Source: CAD feature listing. Evaluate the final solid. Frame: model axes, mm. Coordinates: 2 decimals unless noted, no trailing zeros. Write each loop counter-clockwise with the first axis right and the second up, starting at its lowest first coordinate (ties: lowest second). Pieces come first, ordered by that corner, then holes. Notation, with made-up numbers: M -3.5,-31 L 14.5,-31 A20 ccw 14.5,4 Z; hole C -7.5,85 d5. An arc over 180 degrees is marked long. Write item = value, one per line. Start each with the question number.
1. Section query A-A (y = 581). Output: boundary loops of the cut face in (x, z), then the cut area to 3 significant figures.
2. Section query C-C (x = 26.25). Output: boundary loops of the cut face in (y, z), then the cut area to 3 significant figures.
3. Pin query (flat end, axial travel): pin 1 Ø1.9 at (x, y) = (103.91, 584.08) entering from -Z. Return the tip coordinate at first contact, or that it passes through.
4. Line query: line 1 along X through (y, z) = (573.5, 0.65); line 2 along Y through (x, z) = (26.25, 1.25); line 3 along X through (y, z) = (570, 1.3). Output: solid intervals per line, ascending.
5. Section query D-D (z = 0.4). Output: boundary loops of the cut face in (x, y).
6. Section query B-B (x = 7). Output: boundary loops of the cut face in (y, z).
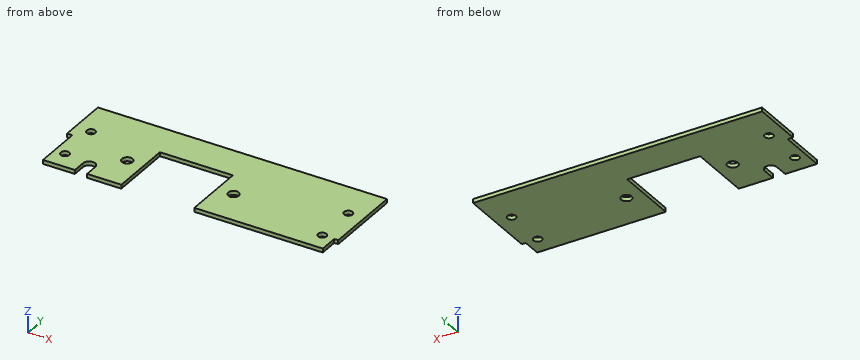
```python
from build123d import *

# Parameters (mm, degrees)
SKETCH1_W           = 110.914742868
SKETCH1_H           = 37
SKETCH1_R           = 1.6
BOSS_EXTRUDE1_DEPTH = 1.5
SKETCH2_W           = 3
SKETCH2_H           = 18
CUT_EXTRUDE1_DEPTH  = 1.5
SKETCH3_W           = 1.5
SKETCH3_H           = 7
SKETCH3_W_2         = 1
SKETCH3_H_2         = 30
SKETCH3_H_3         = 19
CUT_EXTRUDE2_DEPTH  = 10
SKETCH4_R           = 2
SKETCH4_W           = 27.5
SKETCH4_H           = 23.7
CUT_EXTRUDE3_DEPTH  = 10


with BuildPart() as part:
    # Sketch1 → Boss-Extrude1 (new body)
    with BuildSketch(Plane.XY):
        with Locations((55.457371434, 579.580871166)):
            Rectangle(SKETCH1_W, SKETCH1_H)
        with Locations((103.914742868, 584.080871166)):
            Circle(SKETCH1_R, mode=Mode.SUBTRACT)
        with Locations((103.914742868, 568.080871166)):
            Circle(SKETCH1_R, mode=Mode.SUBTRACT)
        with Locations((7, 584.080871166)):
            Circle(SKETCH1_R, mode=Mode.SUBTRACT)
        with Locations((7, 568.080871166)):
            Circle(SKETCH1_R, mode=Mode.SUBTRACT)
    extrude(amount=BOSS_EXTRUDE1_DEPTH)

    # Sketch2 → Cut-Extrude1 (cut)
    with BuildSketch(Plane.XY.offset(1.5)):
        with Locations((1.5, 570.080871166)):
            Rectangle(SKETCH2_W, SKETCH2_H)
    extrude(amount=-CUT_EXTRUDE1_DEPTH, mode=Mode.SUBTRACT)

    # Sketch3 → Cut-Extrude2 (cut)
    with BuildSketch(Plane.XY.offset(1.5)):
        with Locations((109.164742868, 564.580871166)):
            Rectangle(SKETCH3_W, SKETCH3_H)
        with Locations((110.414742868, 564.580871166)):
            Rectangle(SKETCH3_W_2, SKETCH3_H)
        with Locations((110.414742868, 583.080871166)):
            Rectangle(SKETCH3_W_2, SKETCH3_H_2)
        with Locations((0.5, 588.580871166)):
            Rectangle(SKETCH3_W_2, SKETCH3_H_3)
    extrude(amount=-CUT_EXTRUDE2_DEPTH, mode=Mode.SUBTRACT)

    # Sketch4 → Cut-Extrude3 (cut)
    with BuildSketch(Plane.XY.offset(1.5)):
        with Locations((66.25, 574.980871166)):
            Circle(SKETCH4_R)
        with Locations((26.25, 574.980871166)):
            Circle(SKETCH4_R)
        with Locations((46.25, 572.930871166)):
            Rectangle(SKETCH4_W, SKETCH4_H)
        with BuildLine():
            Line((15, 561.080871166), (15, 566.080871166))
            ThreePointArc((15, 566.080871166), (17.3, 568.380871166), (19.6, 566.080871166))
            Line((19.6, 566.080871166), (19.6, 561.080871166))
            ThreePointArc((19.6, 561.080871166), (17.3, 558.780871166), (15, 561.080871166))
        make_face()
    extrude(amount=-CUT_EXTRUDE3_DEPTH, mode=Mode.SUBTRACT)


solid = part.part
```
Results are:
q1.outline = M 1,0 L 32.5,0 L 32.5,1.5 L 1,1.5 Z; M 60,0 L 109.91,0 L 109.91,1.5 L 60,1.5 Z
q1.area = 122 mm^2
q2.outline = M 561.08,0 L 572.98,0 L 572.98,1.5 L 561.08,1.5 Z; M 576.98,0 L 598.08,0 L 598.08,1.5 L 576.98,1.5 Z
q2.area = 49.5 mm^2
q3.pin_1 = through
q4.line_1 = 3 to 24.91, 27.59 to 32.5, 60 to 64.91, 67.59 to 109.91
q4.line_2 = 561.08 to 572.98, 576.98 to 598.08
q4.line_3 = 3 to 32.5, 60 to 109.91
q5.outline = M 1,579.08 L 3,579.08 L 3,561.08 L 15,561.08 L 15,566.08 A2.3 cw 19.6,566.08 L 19.6,561.08 L 32.5,561.08 L 32.5,584.78 L 60,584.78 L 60,561.08 L 108.41,561.08 L 108.41,568.08 L 109.91,568.08 L 109.91,598.08 L 1,598.08 Z; hole C 7,568.08 d3.2; hole C 7,584.08 d3.2; hole C 26.25,574.98 d4; hole C 66.25,574.98 d4; hole C 103.91,568.08 d3.2; hole C 103.91,584.08 d3.2
q6.outline = M 561.08,0 L 566.48,0 L 566.48,1.5 L 561.08,1.5 Z; M 569.68,0 L 582.48,0 L 582.48,1.5 L 569.68,1.5 Z; M 585.68,0 L 598.08,0 L 598.08,1.5 L 585.68,1.5 Z
